Check sheet for the modelled part. Datum: model origin and axes. Units: mm. Face numbers are marked on the shaded views. A direction names the side the tool comes from. Round coordinates to 2 decimals unless told otherwise and drop trailing zeros. Write each loop counter-clockwise with the first axis right and the second up, starting at its lowest first coordinate (ties: lowest second). Pieces come first, ordered by that corner, then holes. Notation, with made-up numbers: M 12,52 L 60,52 A24 cw 60,77 Z; hole C 29,60.25 d8. An arc over 180 degrees is marked long. Answer in a Markdown table with one row per item.
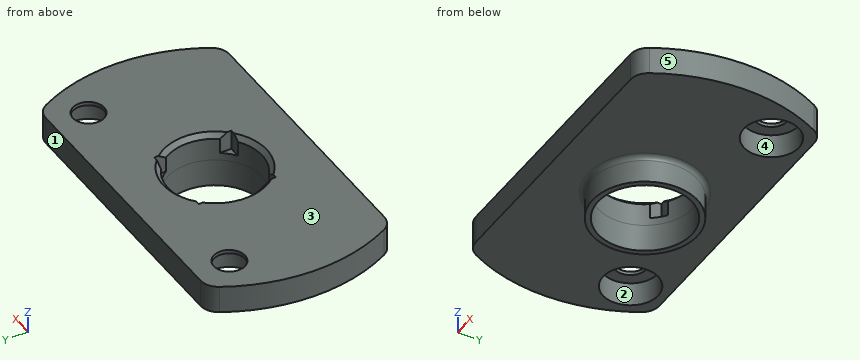
Autodesk Inventor part; units mm, degrees
ref_plane "YZ Plane" through (0, 0, 0) normal (1, 0, 0) x (0, 1, 0)
ref_plane "XZ Plane" through (0, 0, 0) normal (0, 1, 0) x (-1, 0, 0)
ref_plane "XY Plane" through (0, 0, 0) normal (0, 0, 1) x (1, 0, 0)
sketch "Náčrt1" plane through (0, 0, 0) normal (0, 0, 1) x (1, 0, 0)
  circle A0 centre (0, 0) radius 5.125
  arc A1 (8.5, -16.6565) -> (-8.5, -16.6565) centre (0, 0) ccw
  line L0 (-13.35, 6.1) -> (13.35, 6.1)
  line L1 (0, 18.7) -> (0, -18.7)
  line L2 (8.5, -16.6565) -> (8.5, -22.2)
  line L3 (8.5, -22.2) -> (-8.5, -22.2)
  line L4 (-8.5, -22.2) -> (-8.5, -16.6565)
  line L5 (0, -18.7) -> (8.5, -22.2) construction
  line L6 (0, -18.7) -> (-8.5, -22.2) construction
  circle A2 centre (-13.35, 6.1) radius 1.7
  circle A3 centre (13.35, 6.1) radius 1.7
  line L7 (-12.1033, 10) -> (12.1033, 10)
  arc A4 (12.1033, 10) -> (-12.1033, 10) centre (0, 0) ccw
  line L8 (4.2, 4.2) -> (-4.2, 4.2)
  line L9 (-4.2, 4.2) -> (-4.2, -4.2)
  line L10 (-4.2, -4.2) -> (4.2, -4.2)
  line L11 (4.2, -4.2) -> (4.2, 4.2)
  line L12 (4.2, 4.2) -> (-4.2, -4.2) construction
  line L13 (-4.2, 4.2) -> (4.2, -4.2) construction
  line L14 (-3.55, -20.2) -> (3.55, -20.2)
  line L15 (3.55, -20.2) -> (3.55, -17.1)
  line L16 (3.55, -17.1) -> (-3.55, -17.1)
  line L17 (-3.55, -17.1) -> (-3.55, -20.2)
  line L18 (-3.55, -20.2) -> (3.55, -17.1) construction
  line L19 (3.55, -20.2) -> (-3.55, -17.1) construction
  circle A5 centre (0, 0) radius 5.575
  circle A6 centre (0, 0) radius 18.7
  circle A7 centre (-13.35, 6.1) radius 3
  circle A8 centre (13.35, 6.1) radius 3
  line L20 (-17.6407, 10) -> (18.7, 10)
  line L21 (0, 0) -> (-2.6642, 0) construction
  line L22 (-17.6407, -10) -> (18.7, -10)
  point P0 (-10.088, 6.1)
  point P1 (4.2, -2.9369)
  point P2 (2.9369, -4.2)
  point P3 (-2.9369, -4.2)
  point P4 (-4.2, -2.9369)
  point P5 (-4.2, 2.9369)
  point P6 (-2.9369, 4.2)
  point P7 (4.2, 2.9369)
  point P8 (2.9369, 4.2)
  point P9 (0, -18.65)
  point P10 (-8.5, -16.6565)
  point P11 (15.8016, -10)
  point P12 (15.8016, 10)
  point P13 (-15.8016, 10)
  point P14 (-15.8016, -10)
  dimension "d0" = 10.25
  dimension "d1" = 37.4
  dimension "d2" = 26.7
  dimension "d3" = 17
  dimension "d5" = 22.2
  dimension "d7" = 6.1
  dimension "d9" = 3.4
  dimension "d10" = 3.4
  dimension "d12" = 10
  dimension "d14" = 3
  dimension "d25" = 8.4
  dimension "d26" = 8.4
  dimension "d31" = 3.1
  dimension "d32" = 7.1
  dimension "d33" = 2
  dimension "d39" = 0.45
  dimension "d40" = 6
  dimension "d41" = 6
extrude "Vysunutí1" add sketch "Náčrt1" along normal blind 0.4 contours A0 L11 A5 | A0 L8 A5 L11 | L11 A5 L10 A0 | A0 L1 A5 L8 | A5 L8 L11 | L11 L8 A5 L1 L7 L20 A1 L22 L10 | L10 A5 L1 A0 | L11 L10 A5 | A0 L8 A5 L1 | L1 A5 L10 A0 | A0 L9 A5 L8 | A5 L8 L9 L10 L1 L22 A1 L20 L7 | L10 A5 L9 A0 | A0 L9 A5 | A5 L9 L8 | L10 L9 A5 | A7 | A8
extrude "Vysunutí2" add sketch "Náčrt1" against normal blind 2.6 contours A0 L11 A5 | A0 L8 A5 L11 | L11 A5 L10 A0 | A0 L1 A5 L8 | A5 L8 L11 | L11 L8 A5 L1 L7 L20 A1 L22 L10 | L10 A5 L1 A0 | L11 L10 A5 | A0 L8 A5 L1 | L1 A5 L10 A0 | A0 L9 A5 L8 | A5 L8 L9 L10 L1 L22 A1 L20 L7 | L10 A5 L9 A0 | A0 L9 A5 | A5 L9 L8 | L10 L9 A5
chamfer "Zkosení1" distance 0.5 angle 45 1 edges at (-5.125, 0, 0.4)
extrude "Vysunutí3" cut sketch "Náčrt1" along normal blind 0.75 and the other way blind 1.75 contours A0 L8 A5 L11 | L11 A5 L10 A0 | A5 L8 L11 | L11 L10 A5 | A0 L9 A5 L8 | L10 A5 L9 A0 | A5 L9 L8 | L10 L9 A5
sketch "Náčrt2" plane through (0, 0, -2.6) normal (0, 0, -1) x (-1, 0, 0)
  circle A0 centre (0, 0) radius 5.125
  circle A1 centre (0, 0) radius 5.7
  dimension "d35" = 11.4
extrude "Vysunutí4" add sketch "Náčrt2" along normal blind 3
fillet "Zaoblení4" radius 0.5 1 edges at (5.7, 0, -2.6)
fillet "Zaoblení5" radius 2 4 edges at (15.8016, 10, -1.1) (-15.8016, 10, -1.1) (-15.8016, -10, -1.1) (15.8016, -10, -1.1)
properties part number "Držák-Cam+ir V2"
1. Section check D-D, the plane x = 0. Record the cut outline in (y, z) (3 decimals).
Found:
| item | result |
|---|---|
| outline | M -10,-2.6 L -6.2,-2.6 A0.5 cw -5.7,-3.1 L -5.7,-5.6 L -5.125,-5.6 L -5.125,-0.1 L -5.625,0.4 L -10,0.4 Z; M 5.125,-5.6 L 5.7,-5.6 L 5.7,-3.1 A0.5 cw 6.2,-2.6 L 10,-2.6 L 10,0.4 L 5.625,0.4 L 5.125,-0.1 Z |
2. Draft check along Y on the marked faces 3, 4 and 5. Enter one of: +Y half, -Y half, draft (parallel to the pull), parting line (faces both ways), or undercut.
Found:
| item | result |
|---|---|
| face 3 | draft |
| face 4 | undercut |
| face 5 | parting line |
3. Section check A-A, the plane x = 13.35. Record the cut outline in (y, z), and give its area (3 significant figures).
Found:
| item | result |
|---|---|
| outline | M -10,-2.6 L 3.1,-2.6 L 3.1,0 L 4.4,0 L 4.4,0.4 L -10,0.4 Z; M 7.8,0 L 9.1,0 L 9.1,-2.6 L 10,-2.6 L 10,0.4 L 7.8,0.4 Z |
| area | 43.0 mm2 |
4. Scan lines: L1, parallel to Y at x = -13.35, z = 0.25; L2, parallel to Y at x = 0, z = -1.8 (3 decimals); L3, parallel to X at y = 4.25, z = -0.25. Record each from-to range of solid material in increasing order.
Found:
| item | result |
|---|---|
| L1 | y = -10 to 4.4, 7.8 to 10 |
| L2 | y = -10 to -5.125, 5.125 to 10 |
| L3 | x = -18.21 to -15.71, -10.99 to -2.86, 2.86 to 10.99, 15.71 to 18.21 |
5. Section check C-C, the plane z = -1. Record the cut outline in (x, y) (3 decimals), and give its area (3 significant figures).
Found:
| item | result |
|---|---|
| outline | M -16.415,-8.958 A2 ccw -14.659,-10 L 14.659,-10 A2 ccw 16.415,-8.958 A18.7 ccw 16.415,8.958 A2 ccw 14.659,10 L -14.659,10 A2 ccw -16.415,8.958 A18.7 ccw Z; hole C -13.35,6.1 d6; hole M -4.2,-4.2 L -2.937,-4.2 A5.125 ccw 2.937,-4.2 L 4.2,-4.2 L 4.2,-2.937 A5.125 ccw 4.2,2.937 L 4.2,4.2 L 2.937,4.2 A5.125 ccw -2.937,4.2 L -4.2,4.2 L -4.2,2.937 A5.125 ccw -4.2,-2.937 Z; hole C 13.35,6.1 d6 |
| area | 568 mm2 |
6. Section check B-B, the plane y = 0. Record the cut outline in (x, z) (3 decimals), and give its area (3 significant figures).
Found:
| item | result |
|---|---|
| outline | M -18.7,-2.6 L -6.2,-2.6 A0.5 cw -5.7,-3.1 L -5.7,-5.6 L -5.125,-5.6 L -5.125,-0.1 L -5.625,0.4 L -18.7,0.4 Z; M 5.125,-5.6 L 5.7,-5.6 L 5.7,-3.1 A0.5 cw 6.2,-2.6 L 18.7,-2.6 L 18.7,0.4 L 5.625,0.4 L 5.125,-0.1 Z |
| area | 84.8 mm2 |
7. Access from +Z, -Z, +X, -X, +Y, -Y to the whole of each face (thin tool, end or side, straight path). Record for the marked faces 1 and 2.
Found:
| item | result |
|---|---|
| face 1 | +Z, -Z, +X, -X, +Y |
| face 2 | -Z |
8. Go/stop test with flat-tipped pins: pin 1 (6.5 mm diameter, centred on x = 13, y = 6, fed in from -Z); pin 2 (1.4 mm diameter, centred on y = -3.5, z = -1, fed in from +X); pin 3 (3.5 mm diameter, centred on x = -13.35, y = 6.1, fed in from -Z). Record where each tip stops, or that it passes through.
Found:
| item | result |
|---|---|
| pin 1 | stops at z = -2.6 |
| pin 2 | stops at x = 18.49 |
| pin 3 | stops at z = 0 |
